Design review of the part built by this model. Coordinates are the model's own, in mm. Face numbers are marked on the shaded views. A direction names the side the tool comes from. Round coordinates to 2 decimals unless told otherwise and drop trailing zeros. Write each loop counter-clockwise with the first axis right and the second up, starting at its lowest first coordinate (ties: lowest second). Pieces come first, ordered by that corner, then holes. Notation, with made-up numbers: M 56.25,-15 L 78.25,-15 A12 ccw 78.25,0 Z; hole C -28,-39.5 d3. An arc over 180 degrees is marked long. Use CSV: the item, a comma, the result in double quotes.
from build123d import *

# Parameters (mm, degrees)
SCHNITT_LINEAR_AUSTRAGEN1_DEPTH = 5.3


with BuildPart() as part:
    # Skizze1 → Basis-Rotation (revolve)
    with BuildSketch(Plane.XY, mode=Mode.PRIVATE) as basis_rotation_sk:
        Polygon((0, 0), (5, 0), (5, -0.3), (2.5, -2.8), (2.5, -3), (2.0095, -5.25), (2.0095, -20), (0, -20), align=None)
    revolve(basis_rotation_sk.sketch.rotate(Axis((0, 0, 0), (0, -1, 0)), 180), axis=Axis((0, 0, 0), (0, -1, 0)))

    # Skizze2 → Schnitt-Linear austragen1 (cut)
    with BuildSketch(Plane(origin=(0, 0, 0), x_dir=(-1, 0, 0), z_dir=(0, 1, 0))):
        Polygon((0.866025404, -1.5), (-0.866025404, -1.5), (-1.732050808, 0), (-0.866025404, 1.5), (0.866025404, 1.5), (1.732050808, 0), align=None)
    extrude(amount=-SCHNITT_LINEAR_AUSTRAGEN1_DEPTH, mode=Mode.SUBTRACT)


solid = part.part
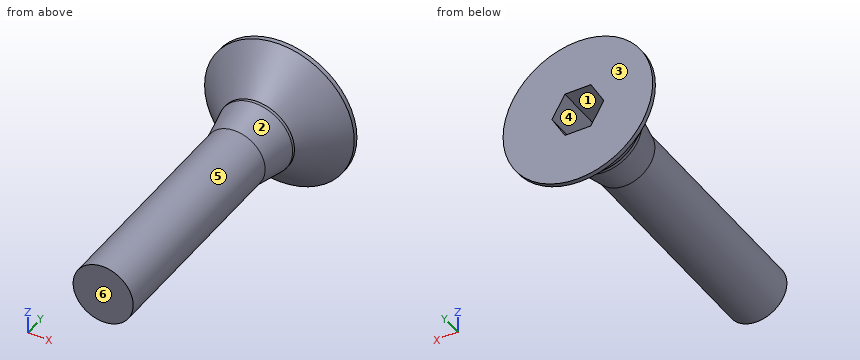
1) Add section B-B on x = 0. Write out the cut boundary in (y, z), then the cut area to 3 significant figures.
Answers:
outline,"M -20,-2.01 L -5.25,-2.01 L -3,-2.5 L -2.8,-2.5 L -0.3,-5 L 0,-5 L 0,-1.5 L -5.3,-1.5 L -5.3,1.5 L 0,1.5 L 0,5 L -0.3,5 L -2.8,2.5 L -3,2.5 L -5.25,2.01 L -20,2.01 Z"
area,"76.3 mm²"
2) The part is to be moulded in two halves that separate along X. For the marked faces 1, 2 and 3, say which applies: released by +X, released by -X, zero draft, split by the parting line, or undercut.
Answers:
face 1,"undercut"
face 2,"split by the parting line"
face 3,"zero draft"
3) Wall thickness on line 1 along Z through (x, y) = (-1.5, -13.25); line 2 along Y through (x, z) = (0, 3.25); line 3 along Z through (x, y) = (2, -3.75): over which ranges is each line inside the solid? List them lowest first. Write a range as [from, to].
Answers:
line 1,"[-1.34, 1.34]"
line 2,"[-2.05, 0]"
line 3,"[-1.21, 1.21]"
4) For pin 1 Ø1.5 at (x, y) = (1.5, -9) entering from +Z; pin 2 Ø0.9 at (x, z) = (0, -0.5) entering from +Y; pin 3 Ø1.9 at (x, y) = (-0.5, -4) entering from +Z, all flat-tipped, find the tip position at first contact; note any pin that passes through.
Answers:
pin 1,"z = 1.86"
pin 2,"y = -5.3"
pin 3,"z = 2.47"
5) Add section A-A on y = -4. Write out the cut boundary in (x, z), then the cut area to 3 significant figures.
Answers:
outline,"C 0,0 d4.56; hole M -1.73,0 L -0.87,-1.5 L 0.87,-1.5 L 1.73,0 L 0.87,1.5 L -0.87,1.5 Z"
area,"8.57 mm²"
6) Machinability: for the marked faces 4, 5 and 6, which of the approach directions +Z, -Z, +X, -X, +Y, -Y give a long, thin tool a straight path to every point of the face, cutting with its end or side? Answer none if there is none.
Answers:
face 4,"+Y"
face 5,"-Y"
face 6,"+Z, -Z, +X, -X, -Y"
7) Add section C-C on y = -11. Write out the cut boundary in (x, z).
Answers:
outline,"C 0,0 d4.02"
